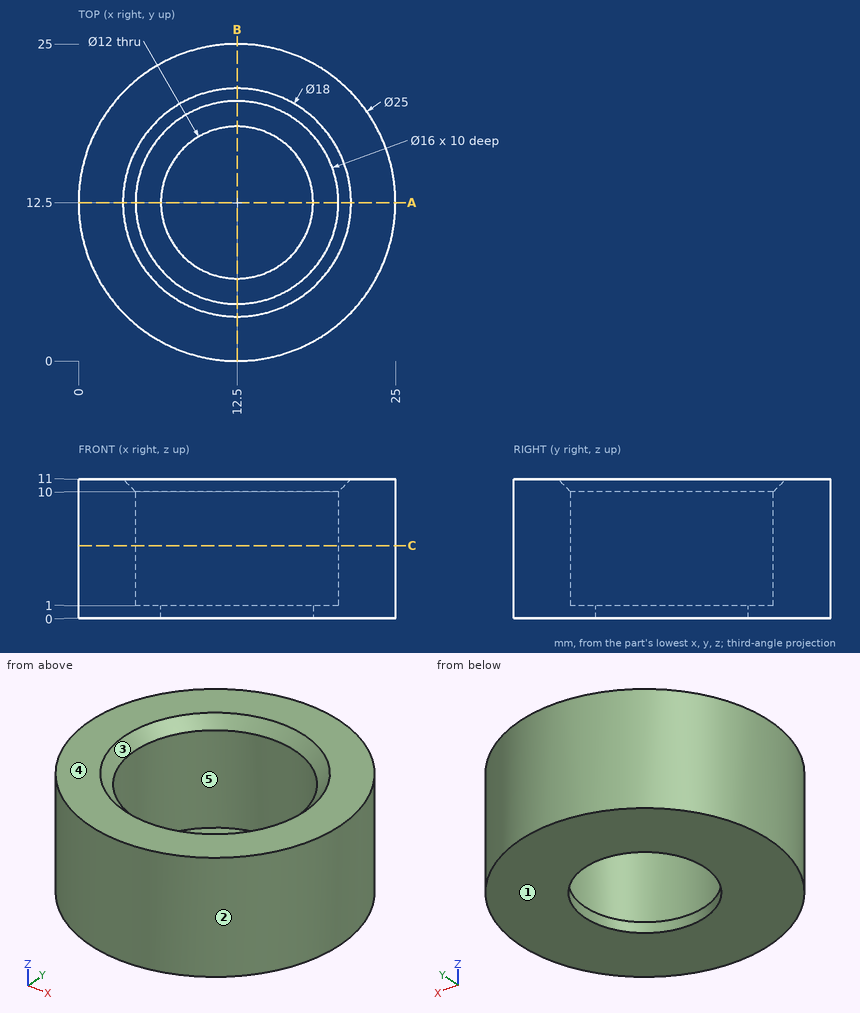
Answer from the drawing. Dimensions are ordinates in mm from the lowest x, y and z of the part. A direction names the side the tool comes from. Coordinates: 2 decimals unless noted, no trailing zeros. Loops run counter-clockwise (first coordinate to the right, second up) from the corner with the lowest first, then second, coordinate; pieces in that order, holes last. Notation, with made-up numbers: (83, 84.5) - (114, 84.5) arc R15 ccw to (114, 102.5) - close; hole circle Ø2 at (-11, -32.75). An arc over 180 degrees is marked (long way). Answer in a Markdown table with one row per item.
1. Find section C-C, the plane z = 5.75. Write down the section's boundary in (x, y).
Conclusion:
| item | result |
|---|---|
| outline | circle Ø25 at (12.5, 12.5); hole circle Ø16 at (12.5, 12.5) |
2. Find section A-A, the plane y = 12.5. Write down the section's boundary in (x, z).
Conclusion:
| item | result |
|---|---|
| outline | (0, 0) - (6.5, 0) - (6.5, 1) - (4.5, 1) - (4.5, 10) - (3.5, 11) - (0, 11) - close; (18.5, 0) - (25, 0) - (25, 11) - (21.5, 11) - (20.5, 10) - (20.5, 1) - (18.5, 1) - close |
3. Straight lines are drawn through the part: line 1 (Y direction, x = 12.5, z = 7); line 2 (Y direction, x = 12.5, z = 0.85); line 3 (X direction, y = 9.75, z = 2). For each, find the intervals that lie inside material, in ascending order.
Conclusion:
| item | result |
|---|---|
| line 1 | y = 0 to 4.5, 20.5 to 25 |
| line 2 | y = 0 to 6.5, 18.5 to 25 |
| line 3 | x = 0.31 to 4.99, 20.01 to 24.69 |
4. Determine the mould class of the marked faces 1, 2 and 3 for opening direction X: +X half, -X half, draft (parallel to the pull), parting line (faces both ways), or undercut.
Conclusion:
| item | result |
|---|---|
| face 1 | draft |
| face 2 | parting line |
| face 3 | undercut |
5. Given pin 1 (1 mm diameter, centred on x = 11.5, z = 6, fed in from -Y); pin 2 (2 mm diameter, centred on x = 16, z = 4.5, fed in from -Y); pin 3 (2 mm diameter, centred on x = 10.5, z = 4, fed in from +Y), each flat-ended and moving along its own axis, determine where each tip first touches the part or whether it passes through.
Conclusion:
| item | result |
|---|---|
| pin 1 | stops at y = 0.01 |
| pin 2 | stops at y = 0.25 |
| pin 3 | stops at y = 24.96 |
6. Which of the six approach directions +Z, -Z, +X, -X, +Y, -Y give full straight-line access (tool end or side, diameter ignored) to the marked faces 4 and 5?
Conclusion:
| item | result |
|---|---|
| face 4 | +Z, +X, -X, +Y, -Y |
| face 5 | +Z |
